Input: part model. Units: mm. Frame: model coordinates. Round coordinates to 2 decimals unless told otherwise and drop trailing zeros. Order: outer loops, then holes, each group sorted by start corner. A loop starts at its lowest first (then second) coordinate and runs counter-clockwise, first axis right, second up. Notation, with made-up numbers: M -38,4 L 15,4 A38 cw 15,43 Z; hole C 13,49 d4. An arc over 180 degrees is marked long. One line per question, with ' | ' between items.
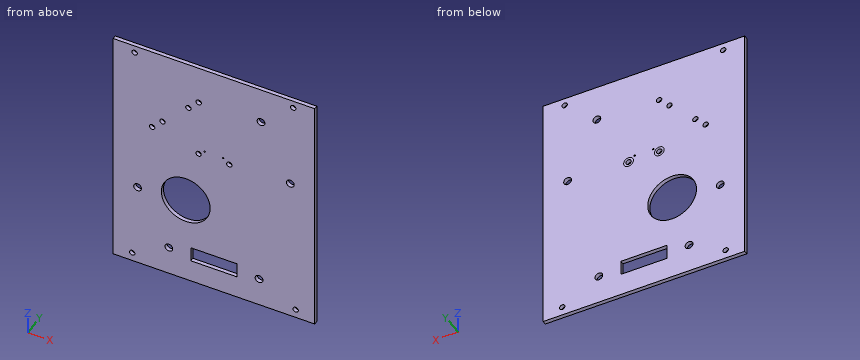
```python
from build123d import *

# Parameters (mm, degrees)
BOSS_EXTRUDE1_DEPTH            = 1.6
F_2_2_2_2_DIAMETER_HOLE1_D     = 2.2
F_2_2_2_2_DIAMETER_HOLE1_DEPTH = 5
SKETCH9_R                      = 10
CUT_EXTRUDE4_DEPTH             = 2.6
SKETCH15_W                     = 83
SKETCH15_H                     = 2.5
CUT_EXTRUDE8_DEPTH             = 2.6
SKETCH37_W                     = 83
SKETCH37_H                     = 1.6
EXTRUDE1_DEPTH                 = 1.6
SKETCH38_W                     = 83
SKETCH38_H                     = 1.6
EXTRUDE2_DEPTH                 = 1.6
F_2_2_2_2_DIAMETER_HOLE4_D     = 2.2
F_2_2_2_2_DIAMETER_HOLE4_DEPTH = 1.6
SKETCH49_W                     = 0.2
SKETCH49_H                     = 100.7
EXTRUDE5_DEPTH                 = 2.6
SKETCH52_W                     = 19
SKETCH52_H                     = 6.1
CUT_EXTRUDE10_DEPTH            = 2.6
SKETCH_2_R                     = 1.6
CUT_EXTRUDE_2_DEPTH            = 10
SKETCH_8_R                     = 0.3
CUT_EXTRUDE_3_DEPTH            = 10
SKETCH_9_R                     = 1.1
CUT_EXTRUDE_4_DEPTH            = 10
SKETCH_10_R                    = 2
CUT_EXTRUDE_5_DEPTH            = 0.01
SKETCH_11_R                    = 1.1
CUT_EXTRUDE_6_DEPTH            = 10


with BuildPart() as part:
    # Sketch1 → Boss-Extrude1 (new body)
    with BuildSketch(Plane(origin=(0, 0, 0), x_dir=(1, 0, 0), z_dir=(0, 1, 0))):
        Polygon((65.24, 0.272495156), (65.24, -46.437452638), (65.24, -63.637452638), (65.24, -70.137452638), (-17.76, -70.137452638), (-17.76, -63.637452638), (-17.76, -48.637452638), (-17.76, -45.78978272), (-17.76, 4.362547362), (-17.76, 21.562547362), (-17.76, 29.862547362), (65.24, 29.862547362), (65.24, 21.562547362), (65.24, 6.562547362), align=None)
    extrude(amount=BOSS_EXTRUDE1_DEPTH)

    # Ø2.2 (2.2) Diameter Hole1
    with Locations(Plane(origin=(0, 1.6, 0), x_dir=(1, 0, 0), z_dir=(0, 1, 0))):
        with Locations((57.24, 27.862547362), (-9.76, 27.862547362)):
            Hole(F_2_2_2_2_DIAMETER_HOLE1_D / 2, depth=F_2_2_2_2_DIAMETER_HOLE1_DEPTH)

    # Sketch9 → Cut-Extrude4 (cut, through all)
    with BuildSketch(Plane(origin=(0, 0, 0), x_dir=(-1, 0, 0), z_dir=(0, -1, 0))):
        with Locations((-12.19, -5.537452638)):
            Circle(SKETCH9_R)
    extrude(amount=-CUT_EXTRUDE4_DEPTH, mode=Mode.SUBTRACT)

    # Sketch15 → Cut-Extrude8 (cut, through all)
    with BuildSketch(Plane.XZ):
        with Locations((23.74, 68.887452638)):
            Rectangle(SKETCH15_W, SKETCH15_H)
    extrude(amount=-CUT_EXTRUDE8_DEPTH, mode=Mode.SUBTRACT)

    # Sketch37 → Extrude1 (add)
    with BuildSketch(Plane(origin=(0, 0, -29.862547362), x_dir=(-1, 0, 0), z_dir=(0, 0, -1))):
        with Locations((-23.74, 0.8)):
            Rectangle(SKETCH37_W, SKETCH37_H)
    extrude(amount=EXTRUDE1_DEPTH)

    # Sketch38 → Extrude2 (add)
    with BuildSketch(Plane.XY.offset(67.637452638)):
        with Locations((23.74, 0.8)):
            Rectangle(SKETCH38_W, SKETCH38_H)
    extrude(amount=EXTRUDE2_DEPTH)

    # Ø2.2 (2.2) Diameter Hole4
    with Locations(Plane(origin=(0, 1.6, 0), x_dir=(1, 0, 0), z_dir=(0, 1, 0))):
        with Locations((-8.76, -66.137452638), (56.24, -66.137452638)):
            Hole(F_2_2_2_2_DIAMETER_HOLE4_D / 2, depth=F_2_2_2_2_DIAMETER_HOLE4_DEPTH)

    # Sketch49 → Extrude5 (cut, through all)
    with BuildSketch(Plane.XZ):
        with Locations((65.14, 18.887452638)):
            Rectangle(SKETCH49_W, SKETCH49_H)
        with Locations((-17.66, 18.887452638)):
            Rectangle(SKETCH49_W, SKETCH49_H)
    extrude(amount=-EXTRUDE5_DEPTH, mode=Mode.SUBTRACT)

    # Sketch52 → Cut-Extrude10 (cut, through all)
    with BuildSketch(Plane.XZ):
        with Locations((23.74, -19.027547362)):
            Rectangle(SKETCH52_W, SKETCH52_H)
    extrude(amount=-CUT_EXTRUDE10_DEPTH, mode=Mode.SUBTRACT)

    # ｽｹｯﾁ2 → ｶｯﾄ - 押し出し2 (cut)
    with BuildSketch(Plane(origin=(0, 0, 0), x_dir=(-1, 0, 0), z_dir=(0, -1, 0))):
        with Locations((-55.04, -30.237452638)):
            Circle(SKETCH_2_R)
        with Locations((7.56, -3.637452638)):
            Circle(SKETCH_2_R)
        with Locations((-42.24, 19.462547362)):
            Circle(SKETCH_2_R)
        with Locations((-5.24, 19.462547362)):
            Circle(SKETCH_2_R)
        with Locations((-43.04, -54.237452638)):
            Circle(SKETCH_2_R)
    extrude(amount=-CUT_EXTRUDE_2_DEPTH, mode=Mode.SUBTRACT)

    # ｽｹｯﾁ8 → ｶｯﾄ - 押し出し3 (cut)
    with BuildSketch(Plane(origin=(0, 1.6, 0), x_dir=(1, 0, 0), z_dir=(0, 1, 0))):
        with Locations((27.54, -31.237452638)):
            Circle(SKETCH_8_R)
        with Locations((19.94, -31.237452638)):
            Circle(SKETCH_8_R)
    extrude(amount=-CUT_EXTRUDE_3_DEPTH, mode=Mode.SUBTRACT)

    # ｽｹｯﾁ9 → ｶｯﾄ - 押し出し4 (cut)
    with BuildSketch(Plane(origin=(0, 1.6, 0), x_dir=(1, 0, 0), z_dir=(0, 1, 0))):
        with Locations((30.04, -29.237452638)):
            Circle(SKETCH_9_R)
        with Locations((17.44, -29.237452638)):
            Circle(SKETCH_9_R)
    extrude(amount=-CUT_EXTRUDE_4_DEPTH, mode=Mode.SUBTRACT)

    # ｽｹｯﾁ10 → ｶｯﾄ - 押し出し5 (cut)
    with BuildSketch(Plane(origin=(0, 1.6, 0), x_dir=(1, 0, 0), z_dir=(0, 1, 0))):
        with Locations((30.04, -29.237452638)):
            Circle(SKETCH_10_R)
        with Locations((17.44, -29.237452638)):
            Circle(SKETCH_10_R)
    extrude(amount=-CUT_EXTRUDE_5_DEPTH, mode=Mode.SUBTRACT)

    # ｽｹｯﾁ11 → ｶｯﾄ - 押し出し6 (cut)
    with BuildSketch(Plane.XZ):
        with Locations((17.512640687, 53.270093325)):
            Circle(SKETCH_11_R)
        with Locations((13.27, 49.027452638)):
            Circle(SKETCH_11_R)
        with Locations((2.66, 38.417452638)):
            Circle(SKETCH_11_R)
        with Locations((-1.587634962, 34.179812111)):
            Circle(SKETCH_11_R)
    extrude(amount=-CUT_EXTRUDE_6_DEPTH, mode=Mode.SUBTRACT)


solid = part.part
```
Item 1: Section query D-D, the plane z = 0. Return loops of the section in (x, y), plus the area to 3 significant figures.
Report:
outline: M -17.56,0 L 3.86,0 L 3.86,1.6 L -17.56,1.6 Z; M 20.52,0 L 65.04,0 L 65.04,1.6 L 20.52,1.6 Z | area: 106 mm²
Item 2: Section query B-B, the plane z = 14. Return loops of the section in (x, y), plus the area to 3 significant figures.
Report:
outline: M -17.56,0 L 6.86,0 L 6.86,1.6 L -17.56,1.6 Z; M 17.52,0 L 65.04,0 L 65.04,1.6 L 17.52,1.6 Z | area: 115 mm²
Item 3: Section query A-A, the plane x = 30.04. Give the number of separate pieces and of enclosed holes in the cut face, plus the area to 3 significant figures.
Report:
separate pieces: 3 | enclosed holes: 0 | area: 148 mm²
Item 4: Line query: line 1 along Z through (x, y) = (23, 0.9); line 2 along X through (y, z) = (0.3, 29); line 3 along Z through (x, y) = (17, 0.7). Output: solid intervals per line, ascending. Write a range as from..to.
Report:
line 1: -31.46..-22.08, -15.98..69.24 | line 2: -17.56..16.37, 18.51..28.97, 31.11..54.03, 56.05..65.04 | line 3: -31.46..-22.08, -15.98..-3.23, 14.3..28.23, 30.25..52.3, 54.24..69.24
Item 5: First-contact query: pin 1 (1.3 mm diameter, centred on x = 57.24, z = -27.86, fed in from -Y); pin 2 (2 mm diameter, centred on x = 30, z = 28.5, fed in from +Y). Flat tips, straight axial feed; report the tip coordinate or a pass-through.
Report:
pin 1: through | pin 2: y = 1.59
